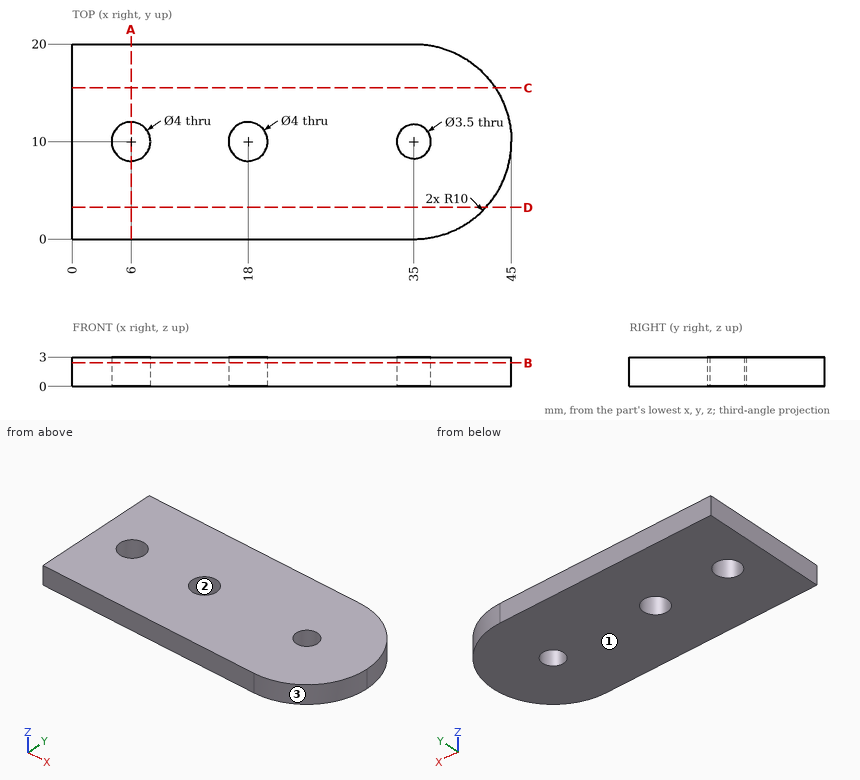
Check sheet for the drawn part. Datum: minimum x, y, z corner. Units: mm. Round coordinates to 2 decimals unless told otherwise and drop trailing zeros. Loops run counter-clockwise (first coordinate to the right, second up) from the corner with the lowest first, then second, coordinate; pieces in that order, holes last. Notation, with made-up numbers: (71, -34) -> (88, -34) arc R20 ccw to (88, -16) -> close; hole circle Ø10 at (15, 75). An arc over 180 degrees is marked (long way). Put each result on its own line as item: value. Start each with the question number.
1. Section check C-C (y = 15.5). Enter the section's corners in (x, z).
2. Draft check along X on the marked faces 1, 2 and 3. Enter one of: +X half, -X half, draft (parallel to the pull), parting line (faces both ways), or undercut.
3. Section check B-B (z = 2.4). Give the number of separate pieces and of enclosed holes in the cut face, plus the area to 3 significant figures.
4. Section check D-D (y = 3.25). Enter the section's corners in (x, z), plus the area to 3 significant figures.
5. Section check A-A (x = 6). Enter the section's corners in (y, z).
6. Scan lines: probe 1 along Y at (x, z) = (18, 1.15); probe 2 along X at (y, z) = (8.75, 1.05) (1 decimal); probe 3 along Y at (x, z) = (35, 1.95). Record each from-to range of solid material in increasing order.
Findings:
1. outline: (0, 0) -> (43.35, 0) -> (43.35, 3) -> (0, 3) -> close
2. face 1: draft
2. face 2: undercut
2. face 3: +X half
3. separate pieces: 1
3. enclosed holes: 3
3. area: 822 mm^2
4. outline: (0, 0) -> (42.38, 0) -> (42.38, 3) -> (0, 3) -> close
4. area: 127 mm^2
5. outline: (0, 0) -> (8, 0) -> (8, 3) -> (0, 3) -> close; (12, 0) -> (20, 0) -> (20, 3) -> (12, 3) -> close
6. probe 1: y = 0 to 8, 12 to 20
6. probe 2: x = 0 to 4.4, 7.6 to 16.4, 19.6 to 33.8, 36.2 to 44.9
6. probe 3: y = 0 to 8.25, 11.75 to 20
